For this review, take the finished solid that the model builds, in its own axes (mm). A direction names the side the tool comes from. Coordinates: 2 decimals unless noted, no trailing zeros. Loops run counter-clockwise (first coordinate to the right, second up) from the corner with the lowest first, then second, coordinate; pieces in that order, holes last. Notation, with made-up numbers: (-1.75, 31.25) -> (26.25, 31.25) arc R19 ccw to (26.25, 63.25) -> close; hole circle Ø9 at (35, 29). An arc over 180 degrees is marked (long way). Answer in a Markdown table with one row per item.
from build123d import *

# Parameters (mm, degrees)
SKETCH3_R               = 8
BOSS_EXTRUDE1_DEPTH     = 20
SKETCH4_R               = 4
CUT_EXTRUDE1_DEPTH      = 12
CUT_EXTRUDE2_DEPTH      = 23.978250586
CUT_EXTRUDE2_DEPTH_BACK = 23.978250586
SKETCH5_R               = 1.5
SKETCH6_W               = 5.7
SKETCH6_H               = 4
CUT_EXTRUDE3_DEPTH      = 6


with BuildPart() as part:
    # Sketch3 → Boss-Extrude1 (new body)
    with BuildSketch(Plane(origin=(0, 0, 0), x_dir=(1, 0, 0), z_dir=(0, 1, 0))):
        with Locations(Location((0, 0, 0), (0, 0, 270))):
            Circle(SKETCH3_R)
    extrude(amount=BOSS_EXTRUDE1_DEPTH)

    # Sketch4 → Cut-Extrude1 (cut)
    with BuildSketch(Plane.XZ):
        with Locations(Location((0, 0, 0), (0, 0, 270))):
            Circle(SKETCH4_R)
    extrude(amount=-CUT_EXTRUDE1_DEPTH, mode=Mode.SUBTRACT)

    # Sketch5 → Cut-Extrude2 (cut, two sides: drawn at the far end of the back side and taken through both)
    with BuildSketch(Plane(origin=(0, 0, 0), x_dir=(0, 0, -1), z_dir=(1, 0, 0)).offset(-CUT_EXTRUDE2_DEPTH_BACK)):
        with Locations((0, 2.5)):
            Circle(SKETCH5_R)
    extrude(amount=CUT_EXTRUDE2_DEPTH + CUT_EXTRUDE2_DEPTH_BACK, mode=Mode.SUBTRACT)

    # Sketch6 → Cut-Extrude3 (cut)
    with BuildSketch(Plane(origin=(0, 20, 0), x_dir=(1, 0, 0), z_dir=(0, 1, 0))):
        with Locations((-0.034439742, -0.098165146)):
            Rectangle(SKETCH6_W, SKETCH6_H)
    extrude(amount=-CUT_EXTRUDE3_DEPTH, mode=Mode.SUBTRACT)


solid = part.part
Item 1: The part is to be moulded in two halves that separate along X. For faces 4 (the cylindrical face through (-7.81, 9.86, -1.73)), 5 (the flat face through (-2, 0, -4)), 6 (the flat face through (2.816, 17, 0)), say which applies: +X half, -X half, draft (parallel to the pull), parting line (faces both ways), or undercut.
Worked answers:
| item | result |
|---|---|
| face 4 | parting line |
| face 5 | draft |
| face 6 | undercut |
Item 2: For faces 1 (the cylindrical face through (-5.886, 1.925, -1.386)), 2 (the flat face through (0, 12, 0)), 3 (the flat face through (0, 17, -1.902)), list the 3-axis set-ups (+Z, -Z, +X, -X, +Y, -Y) from which the entire face can be reached by the end or side of a thin tool; tool diameter is ignored.
Worked answers:
| item | result |
|---|---|
| face 1 | +X, -X |
| face 2 | -Y |
| face 3 | +Y |
Item 3: Insertion check: pin 1 (4 mm diameter, centred on x = -1, z = -1.5, fed in from -Y); pin 2 (6 mm diameter, centred on x = 3.5, y = 17, fed in from -Z); pin 3 (1 mm diameter, centred on x = -3, y = 2.5, fed in from -Z); pin 4 (2.5 mm diameter, centred on y = 2.5, z = 0, fed in from +X). Each pin has a flat end and moves straight along its axis. Give the tip position at first contact, or say it passes through.
Worked answers:
| item | result |
|---|---|
| pin 1 | y = 12 |
| pin 2 | z = -7.98 |
| pin 3 | z = -7.6 |
| pin 4 | through |
Item 4: Take a section at A-A, the plane z = 0. State the section outline as (x, y) points.
Worked answers:
| item | result |
|---|---|
| outline | (-8, 0) -> (-4, 0) -> (-4, 1) -> (-8, 1) -> close; (-8, 4) -> (-4, 4) -> (-4, 12) -> (4, 12) -> (4, 4) -> (8, 4) -> (8, 20) -> (2.82, 20) -> (2.82, 14) -> (-2.88, 14) -> (-2.88, 20) -> (-8, 20) -> close; (4, 0) -> (8, 0) -> (8, 1) -> (4, 1) -> close |
Item 5: Take a section at C-C, the plane x = 0. State the section outline as (y, z) points, and give its area (3 significant figures).
Worked answers:
| item | result |
|---|---|
| outline | (0, -8) -> (20, -8) -> (20, -1.9) -> (14, -1.9) -> (14, 2.1) -> (20, 2.1) -> (20, 8) -> (0, 8) -> (0, 4) -> (12, 4) -> (12, -4) -> (0, -4) -> close |
| area | 200 mm² |
Item 6: Take a section at D-D, the plane y = 2.5. State the section outline as (x, z) points, and give its area (3 significant figures).
Worked answers:
| item | result |
|---|---|
| outline | (-7.86, -1.5) arc R8 ccw to (7.86, -1.5) -> (3.71, -1.5) arc R4 cw to (-3.71, -1.5) -> close; (-7.86, 1.5) -> (-3.71, 1.5) arc R4 cw to (3.71, 1.5) -> (7.86, 1.5) arc R8 ccw to start |
| area | 127 mm² |
Item 7: Take a section at B-B, the plane y = 14.25. State the section outline as (x, z) points.
Worked answers:
| item | result |
|---|---|
| outline | circle Ø16 at (0, 0); hole (-2.88, -1.9) -> (2.82, -1.9) -> (2.82, 2.1) -> (-2.88, 2.1) -> close |
Item 8: For L1, parallel to Y at x = -4.75, z = 0; L2, parallel to X at y = 9.25, z = 0; L3, parallel to Y at x = -3, z = -2.5, list the stretches that pass through material, from the lowest coordinate up.
Worked answers:
| item | result |
|---|---|
| L1 | 0 to 1, 4 to 20 |
| L2 | -8 to -4, 4 to 8 |
| L3 | 12 to 20 |
